Source: three-view drawing plus pictorial views. Frame: mm from the lowest corner of the part. Give positions to 0.01 mm unless a question says otherwise; leave off trailing zeros. Loops run counter-clockwise (first coordinate to the right, second up) from the corner with the lowest first, then second, coordinate; pieces in that order, holes last. Notation, with made-up numbers: (9.25, -21.75) - (52.25, -21.75) arc R9 cw to (52.25, -10.75) - close; hole circle Ø10 at (51, 20). An arc over 180 degrees is marked (long way). Answer as a JSON object with one key per item and string values. Group by question number.
(1) Material intervals for L1, parallel to Z at x = 10, y = 7.25; L2, parallel to Z at x = 26.25, y = 1.5; L3, parallel to X at y = 4.15, z = 47, sorted ascending.
(2) Section query D-D (x = 27). Return loops of the section in (y, z).
(3) Pin query (flat end, axial travel): P1, Ø1.6, axis at y = 7.5, z = 28.5, coming from the +X side; P2, Ø1.5, axis at y = 3, z = 7, coming from the +X side; P3, Ø3, axis at x = 25.5, y = 2, coming from the +Z side; P4, Ø7.5, axis at x = 12, z = 29.5, coming from the -Y side. Return the tip coordinate at first contact, or that it passes through.
(4) Section query B-B (z = 10). Return loops of the section in (x, y).
(5) Section query C-C (x = 10). Return loops of the section in (y, z).
(6) Section query A-A (y = 4.15). Return loops of the section in (x, z).
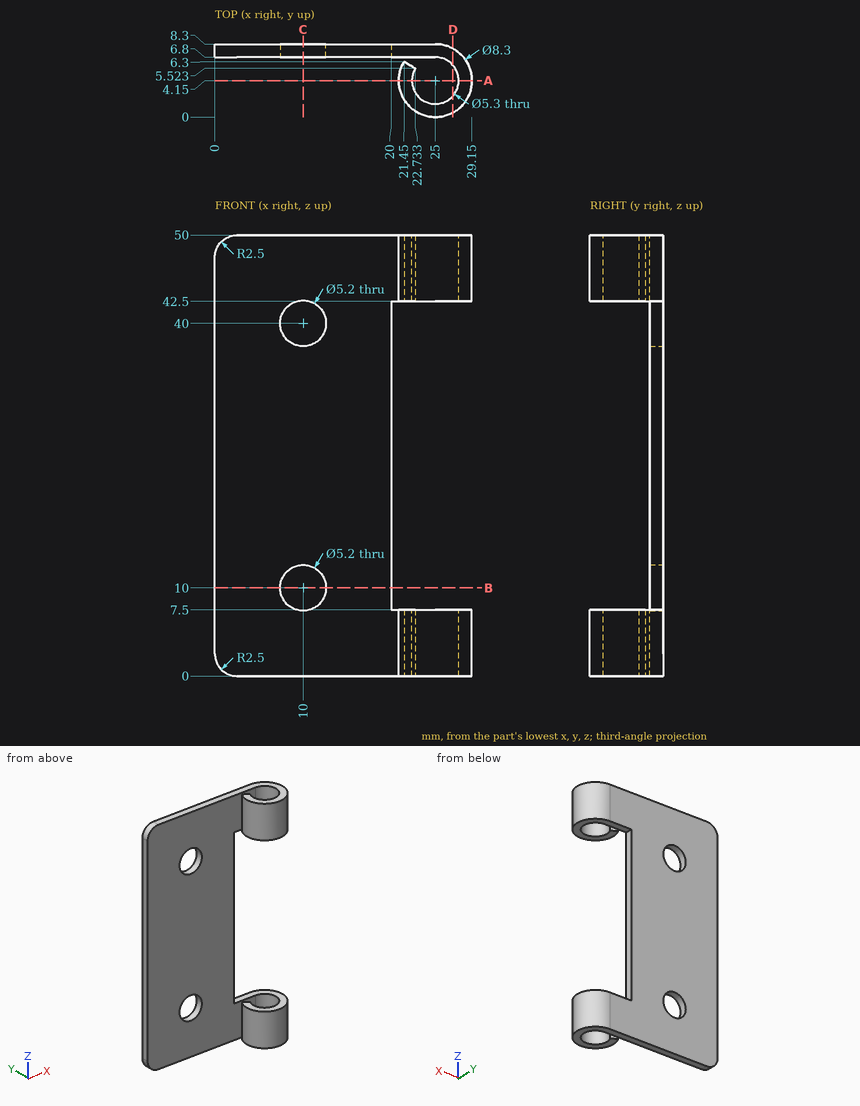
Recorded:
{
 "1": {"L1": "z = 0 to 7.4, 12.6 to 37.4, 42.6 to 50", "L2": "z = 0 to 7.5, 42.5 to 50", "L3": "x = 20.85 to 22.35, 27.65 to 29.15"},
 "2": {"outline": "(0.51, 0) - (2.41, 0) - (2.41, 7.5) - (0.51, 7.5) - close; (0.51, 42.5) - (2.41, 42.5) - (2.41, 50) - (0.51, 50) - close; (5.89, 0) - (7.79, 0) - (7.79, 7.5) - (5.89, 7.5) - close; (5.89, 42.5) - (7.79, 42.5) - (7.79, 50) - (5.89, 50) - close"},
 "3": {"P1": "stops at x = 20", "P2": "stops at x = 29.13", "P3": "stops at z = 50", "P4": "stops at y = 6.8"},
 "4": {"outline": "(0, 6.8) - (7.4, 6.8) - (7.4, 8.3) - (0, 8.3) - close; (12.6, 6.8) - (20, 6.8) - (20, 8.3) - (12.6, 8.3) - close"},
 "5": {"outline": "(6.8, 0) - (8.3, 0) - (8.3, 7.4) - (6.8, 7.4) - close; (6.8, 12.6) - (8.3, 12.6) - (8.3, 37.4) - (6.8, 37.4) - close; (6.8, 42.6) - (8.3, 42.6) - (8.3, 50) - (6.8, 50) - close"},
 "6": {"outline": "(20.85, 0) - (22.35, 0) - (22.35, 7.5) - (20.85, 7.5) - close; (20.85, 42.5) - (22.35, 42.5) - (22.35, 50) - (20.85, 50) - close; (27.65, 0) - (29.15, 0) - (29.15, 7.5) - (27.65, 7.5) - close; (27.65, 42.5) - (29.15, 42.5) - (29.15, 50) - (27.65, 50) - close"}
}
